Build history of the part. All positions in model axes, mm. Face numbers are marked on the shaded views. Give positions to 0.01 mm unless a question says otherwise; leave off trailing zeros. Loops run counter-clockwise (first coordinate to the right, second up) from the corner with the lowest first, then second, coordinate; pieces in that order, holes last. Notation, with made-up numbers: (28, 29.25) -> (38, 29.25) arc R18 ccw to (38, 61.25) -> close; hole circle Ø4 at (65.5, 64.5). An arc over 180 degrees is marked (long way). One line per question, with ' | ' between items. Start each with the question number.
(1) Slice it at B-B, the plane x = 76.2. Write the cut outline in (y, z), then the cut area to 3 significant figures.
(2) Drill centre lines: L1, parallel to Y at x = 57, z = 30.5; L2, parallel to Y at x = 76.2, z = 46. Where is each one in solid material? Low to high. Write a range as from..to.
(3) Flat gauge pin, fed straight in: pin 1 Ø11.5 at (x, z) = (93.5, 17.5) entering from -Y. Where does the tip first touch, or does it go through?
(4) Slice it at C-C, the plane y = 127. Write the cut outline in (x, z).
(5) Slice it at D-D, the plane y = 56.5. Write the cut outline in (x, z), then the cut area to 3 significant figures.
(6) Slice it at A-A, the plane z = 31.5. Write the cut outline in (x, y).
(7) Mould opens along Y. For the marked faces 1, 2, 3 and 4 say: pulls with the +Y half, pulls with the -Y half, needs draft (parallel to the pull), parting line crosses it, or undercut.
```python
from build123d import *

# Parameters (mm, degrees)
F0_W     = 152.4
F0_H     = 152.4
F0_W_2   = 50.8
F0_H_2   = 50.8
F1_DEPTH = 50.8
F2_T     = -6.35
F3_W     = 6.35
F3_H     = 38.1
F4_DEPTH = 139.7
F5_W     = 152.4
F5_H     = 152.4
F6_DEPTH = 12.7
F7_R     = 7.14375
F8_DEPTH = 76.2


with BuildPart() as f1:
    # F0 (on Top) → F1 (new body)
    with BuildSketch(Plane.XY):
        with Locations((76.2, 76.2)):
            Rectangle(F0_W, F0_H)
        with Locations((76.2, 76.2)):
            Rectangle(F0_W_2, F0_H_2, mode=Mode.SUBTRACT)
    extrude(amount=F1_DEPTH)

    # F2
    f2_openings = [f1.faces().sort_by_distance(p)[0] for p in [
        (76.2, 0, 25.4),
    ]]
    offset(amount=F2_T, openings=f2_openings, kind=Kind.INTERSECTION)

    # F3 (on face) → F4 (join)
    with BuildSketch(Plane.YZ.offset(6.35)):
        with Locations((3.175, 25.4)):
            Rectangle(F3_W, F3_H)
    extrude(amount=F4_DEPTH)

    # F5 (on face) → F6 (join)
    with BuildSketch(Plane(origin=(0, 0, 0), x_dir=(1, 0, 0), z_dir=(0, 0, -1))):
        with Locations((76.2, -76.2)):
            Rectangle(F5_W, F5_H)
    extrude(amount=F6_DEPTH)

    # F7 (on face) → F8 (cut)
    with BuildSketch(Plane.XY.offset(50.8)):
        with Locations((76.2, 127)):
            Circle(F7_R)
    extrude(amount=-F8_DEPTH, mode=Mode.SUBTRACT)


solid = f1.part
```
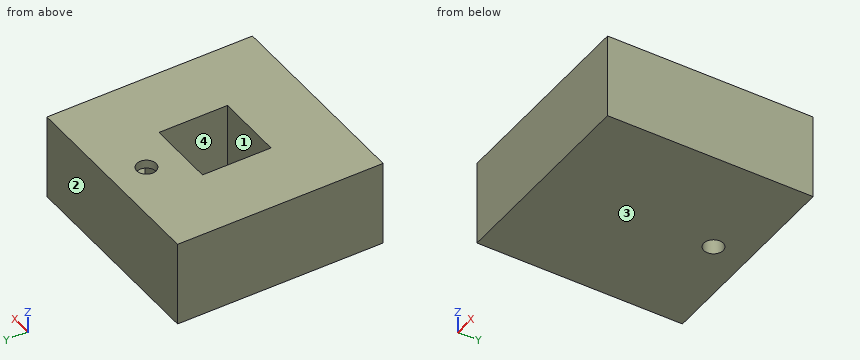
Final values:
1) outline: (0, -12.7) -> (119.86, -12.7) -> (119.86, 6.35) -> (107.95, 6.35) -> (107.95, 44.45) -> (119.86, 44.45) -> (119.86, 50.8) -> (101.6, 50.8) -> (101.6, 0) -> (50.8, 0) -> (50.8, 50.8) -> (0, 50.8) -> close; (134.14, -12.7) -> (152.4, -12.7) -> (152.4, 50.8) -> (134.14, 50.8) -> (134.14, 44.45) -> (146.05, 44.45) -> (146.05, 6.35) -> (134.14, 6.35) -> close; hole (6.35, 6.35) -> (44.45, 6.35) -> (44.45, 44.45) -> (6.35, 44.45) -> close | area: 3,830 mm2
2) L1: 0..6.35, 44.45..50.8, 101.6..107.95, 146.05..152.4 | L2: 0..50.8, 101.6..119.86, 134.14..152.4
3) pin 1: y = 0
4) outline: (0, -12.7) -> (69.06, -12.7) -> (69.06, 6.35) -> (6.35, 6.35) -> (6.35, 44.45) -> (69.06, 44.45) -> (69.06, 50.8) -> (0, 50.8) -> close; (83.34, -12.7) -> (152.4, -12.7) -> (152.4, 50.8) -> (83.34, 50.8) -> (83.34, 44.45) -> (146.05, 44.45) -> (146.05, 6.35) -> (83.34, 6.35) -> close
5) outline: (0, -12.7) -> (152.4, -12.7) -> (152.4, 50.8) -> (101.6, 50.8) -> (101.6, 0) -> (50.8, 0) -> (50.8, 50.8) -> (0, 50.8) -> close; hole (6.35, 6.35) -> (44.45, 6.35) -> (44.45, 44.45) -> (6.35, 44.45) -> close; hole (107.95, 6.35) -> (146.05, 6.35) -> (146.05, 44.45) -> (107.95, 44.45) -> close | area: 4,190 mm2
6) outline: (0, 0) -> (152.4, 0) -> (152.4, 152.4) -> (0, 152.4) -> close; (44.45, 44.45) -> (107.95, 44.45) -> (107.95, 107.95) -> (44.45, 107.95) -> close; hole (6.35, 6.35) -> (146.05, 6.35) -> (146.05, 146.05) -> (6.35, 146.05) -> close; hole (50.8, 50.8) -> (101.6, 50.8) -> (101.6, 101.6) -> (50.8, 101.6) -> close
7) face 1: undercut | face 2: pulls with the +Y half | face 3: needs draft | face 4: undercut
